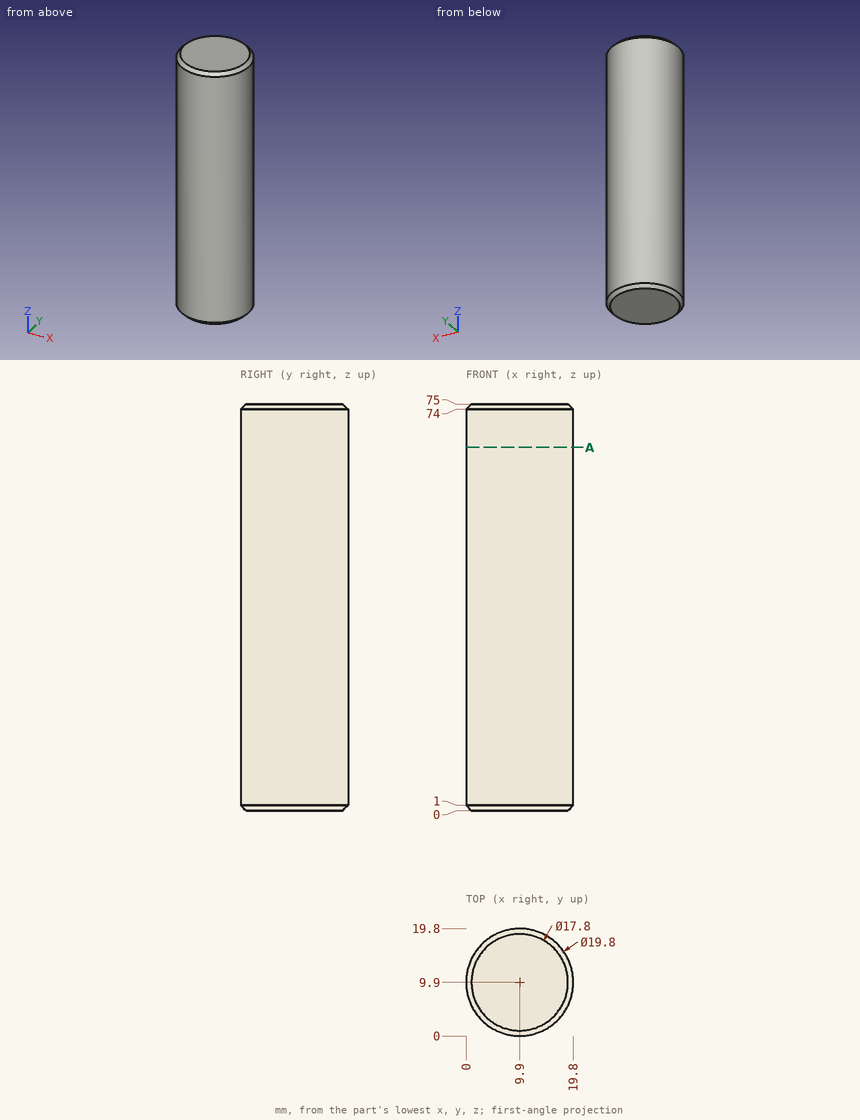
Can you work these out from the drawing? Everything is in mm from the part's minimum corner. Coordinates: 2 decimals unless noted, no trailing zeros. Loops run counter-clockwise (first coordinate to the right, second up) from the corner with the lowest first, then second, coordinate; pieces in that order, holes last. Notation, with made-up numbers: (7.5, -2) -> (43.5, -2) arc R30 ccw to (43.5, 30) -> close; hole circle Ø1 at (17, 25). An arc over 180 degrees is marked (long way). Return JSON: item names as keys, results as strings.
1) Will these pins go through, and if not, where does the flat tip stop? pin 1 (3 mm diameter, centred on x = 7, z = 59, fed in from +Y); pin 2 (1 mm diameter, centred on x = 15.5, z = 45.5, fed in from -Y); pin 3 (6 mm diameter, centred on y = 4, z = 50.5, fed in from +X).
Results below:
{"pin 1": "y = 19.7", "pin 2": "y = 1.41", "pin 3": "x = 19.37"}
2) I need wall thicknesses on line 1 (X direction, y = 9.5, z = 47.5); line 2 (Y direction, x = 18, z = 29); line 3 (Y direction, x = 7.5, z = 39). Which ranges of each line are inside material? Lowest first, please. Write a range as from..to.
Results below:
{"line 1": "0.01..19.79", "line 2": "4.21..15.59", "line 3": "0.3..19.5"}
3) If we section it at A-A, the plane z = 67: Write out the boundary of the cut face in (x, y).
Results below:
{"outline": "circle Ø19.8 at (9.9, 9.9)"}
